```python
from build123d import *

# Parameters (mm, degrees)
SKETCH1_W           = 609.6
SKETCH1_H           = 609.6
BOSS_EXTRUDE1_DEPTH = 3.175
CUT_EXTRUDE2_DEPTH  = 432.063986695
CUT_EXTRUDE3_DEPTH  = 432.063986695


with BuildPart() as part:
    # Sketch1 → Boss-Extrude1 (new body)
    with BuildSketch(Plane(origin=(0, 0, 0), x_dir=(1, 0, 0), z_dir=(0, 1, 0))):
        Rectangle(SKETCH1_W, SKETCH1_H)
    extrude(amount=BOSS_EXTRUDE1_DEPTH)

    # Sketch3 → Cut-Extrude2 (cut, through all)
    with BuildSketch(Plane(origin=(0, 3.175, 0), x_dir=(1, 0, 0), z_dir=(0, 1, 0))):
        with BuildLine():
            Line((-31.060660172, -28.939339828), (28.939339828, 31.060660172))
            ThreePointArc((28.939339828, 31.060660172), (31.060660172, 31.060660172), (31.060660172, 28.939339828))
            Line((31.060660172, 28.939339828), (-28.939339828, -31.060660172))
            ThreePointArc((-28.939339828, -31.060660172), (-31.060660172, -31.060660172), (-31.060660172, -28.939339828))
        make_face()
    extrude(amount=-CUT_EXTRUDE2_DEPTH, mode=Mode.SUBTRACT)

    # Sketch4 → Cut-Extrude3 (cut, through all)
    with BuildSketch(Plane(origin=(0, 3.175, 0), x_dir=(1, 0, 0), z_dir=(0, 1, 0))):
        with BuildLine():
            Line((-50, -1.5), (-120, -1.5))
            ThreePointArc((-120, -1.5), (-121.5, 0), (-120, 1.5))
            Line((-120, 1.5), (-50, 1.5))
            ThreePointArc((-50, 1.5), (-48.5, 0), (-50, -1.5))
        make_face()
        with BuildLine():
            Line((-1.5, 50), (-1.5, 120))
            ThreePointArc((-1.5, 120), (0, 121.5), (1.5, 120))
            Line((1.5, 120), (1.5, 50))
            ThreePointArc((1.5, 50), (0, 48.5), (-1.5, 50))
        make_face()
        with BuildLine():
            Line((-1.5, -275), (-1.5, -205))
            ThreePointArc((-1.5, -205), (0, -203.5), (1.5, -205))
            Line((1.5, -205), (1.5, -275))
            ThreePointArc((1.5, -275), (0, -276.5), (-1.5, -275))
        make_face()
        with BuildLine():
            Line((275, -1.5), (115, -1.5))
            ThreePointArc((115, -1.5), (113.5, 0), (115, 1.5))
            Line((115, 1.5), (275, 1.5))
            ThreePointArc((275, 1.5), (276.5, 0), (275, -1.5))
        make_face()
        with BuildLine():
            Line((-275, 1.5), (-205, 1.5))
            ThreePointArc((-205, 1.5), (-203.5, 0), (-205, -1.5))
            Line((-205, -1.5), (-275, -1.5))
            ThreePointArc((-275, -1.5), (-276.5, 0), (-275, 1.5))
        make_face()
        with BuildLine():
            Line((1.5, 275), (1.5, 205))
            ThreePointArc((1.5, 205), (0, 203.5), (-1.5, 205))
            Line((-1.5, 205), (-1.5, 275))
            ThreePointArc((-1.5, 275), (0, 276.5), (1.5, 275))
        make_face()
    extrude(amount=-CUT_EXTRUDE3_DEPTH, mode=Mode.SUBTRACT)


solid = part.part
```
Part model, mm, in its own coordinate system. A direction names the side the tool comes from. Round coordinates to 2 decimals unless told otherwise and drop trailing zeros. One line per question, with ' | ' between items.
(1) Two-plate mould, pull along Z, no slides. Class faces 1 (the face through (1.48, 1.61, 0.64)), 2 (the face through (-4, 3.175, -4)): released by +Z, released by -Z, zero draft, split by the parting line, or undercut.
Answer key:
face 1: undercut | face 2: zero draft
(2) 3-axis set-ups, long thin cutter, end or side, ignore diameter. For faces 3 (the face through (-1.48, 1.61, -0.64)), 4 (the face through (-4, 0, -4)): which of +Z, -Z, +X, -X, +Y, -Y reach the whole face in a straight line?
Answer key:
face 3: +Y, -Y | face 4: +Z, -Z, +X, -X, -Y
(3) Probe line 1 along X through (y, z) = (0.9, -31); line 2 along Z through (x, y) = (-235.5, 0.25). List the from-to ranges inside material, lowest first.
Answer key:
line 1: x = -304.8 to 28.88, 31.12 to 304.8 | line 2: z = -304.8 to -1.5, 1.5 to 304.8
